Print and shaded views of the part. All mm, measured from the part's lowest x, y and z. Give positions to 0.01 mm unless a question says otherwise; leave off trailing zeros. Loops run counter-clockwise (first coordinate to the right, second up) from the corner with the lowest first, then second, coordinate; pieces in that order, holes last. Notation, with made-up numbers: M -15,66 L 37,66 A36 ccw 37,100 Z; hole C 46.25,86 d6. An arc over 180 degrees is marked long. Answer in a Markdown table with one row per item.
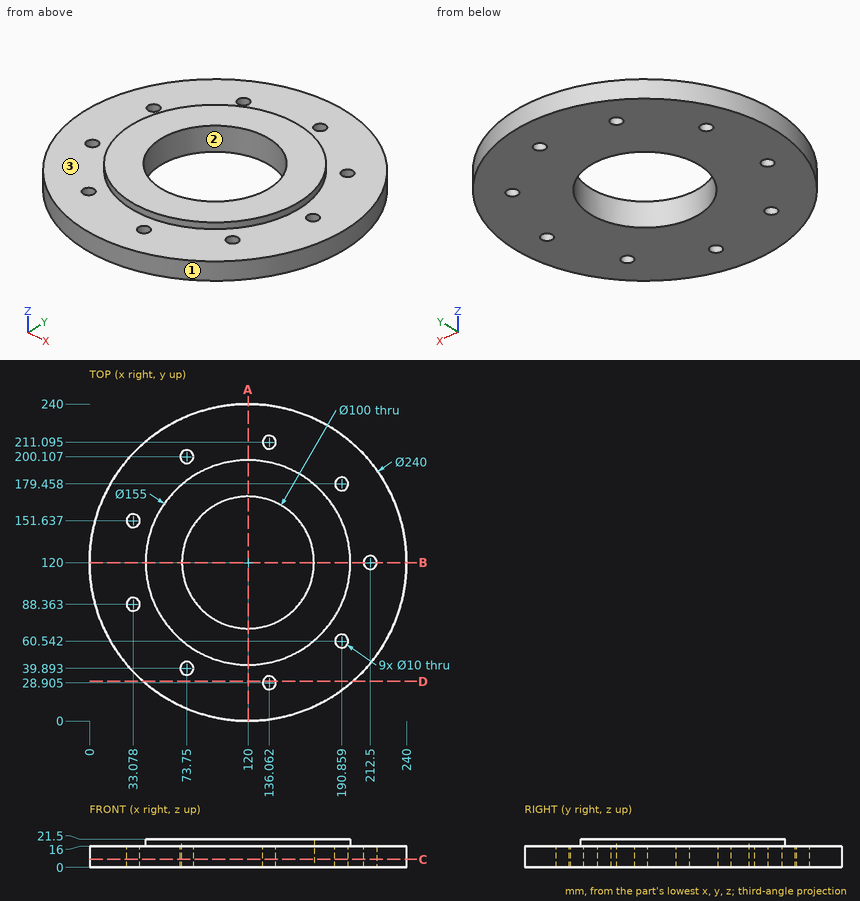
(1) Saw through at B-B, the plane y = 120. Give the cut face in (x, z), and give its area (3 significant figures).
Established:
| item | result |
|---|---|
| outline | M 0,0 L 70,0 L 70,21.5 L 42.5,21.5 L 42.5,16 L 0,16 Z; M 170,0 L 207.5,0 L 207.5,16 L 197.5,16 L 197.5,21.5 L 170,21.5 Z; M 217.5,0 L 240,0 L 240,16 L 217.5,16 Z |
| area | 2,380 mm2 |
(2) Flat gauge pins, fed straight in: P1, Ø16, axis at x = 33.08, y = 88.36, coming from the +Z side; P2, Ø1, axis at y = 137.5, z = 9, coming from the -X side; P3, Ø10, axis at y = 77.5, z = 10, coming from the -X side. Where does each tip first touch, or does it go through?
Established:
| item | result |
|---|---|
| P1 | stops at z = 16 |
| P2 | stops at x = 1.21 |
| P3 | stops at x = 6.01 |
(3) Saw through at C-C, the plane z = 6. Count the separate pieces of the cut face and the enclosed holes in it, and give its area (3 significant figures).
Established:
| item | result |
|---|---|
| separate pieces | 1 |
| enclosed holes | 10 |
| area | 36,700 mm2 |
(4) Wall check: L1, parallel to X at y = 120.5, z = 3.5 (1 decimal); L2, parallel to Y at x = 189.5, z = 15 (1 decimal); L3, parallel to Y at x = 73.75, z = 12.5 (1 decimal). Give the ranges that are in metal, low to high.
Established:
| item | result |
|---|---|
| L1 | x = 0 to 70, 170 to 207.5, 217.5 to 240 |
| L2 | y = 22.2 to 55.7, 65.4 to 174.6, 184.3 to 217.8 |
| L3 | y = 9.3 to 34.9, 44.9 to 101, 139 to 195.1, 205.1 to 230.7 |
(5) Saw through at D-D, the plane y = 30. Give the cut face in (x, z), and give its area (3 significant figures).
Established:
| item | result |
|---|---|
| outline | M 40.63,0 L 131.18,0 L 131.18,16 L 40.63,16 Z; M 140.94,0 L 199.37,0 L 199.37,16 L 140.94,16 Z |
| area | 2,380 mm2 |
(6) Saw through at A-A, the plane x = 120. Give the cut face in (y, z), and give its area (3 significant figures).
Established:
| item | result |
|---|---|
| outline | M 0,0 L 70,0 L 70,21.5 L 42.5,21.5 L 42.5,16 L 0,16 Z; M 170,0 L 240,0 L 240,16 L 197.5,16 L 197.5,21.5 L 170,21.5 Z |
| area | 2,540 mm2 |
(7) Mould opens along X. For the marked faces 1, 2 and 3 say: pulls with the +X half, pulls with the -X half, needs draft (parallel to the pull), parting line crosses it, or undercut.
Established:
| item | result |
|---|---|
| face 1 | parting line crosses it |
| face 2 | undercut |
| face 3 | needs draft |
